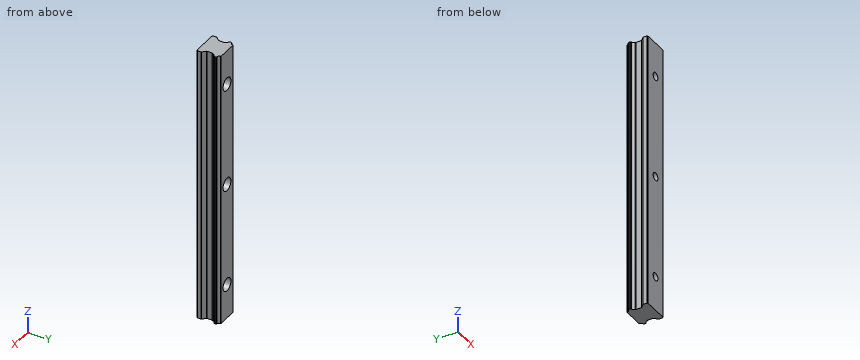
Autodesk Inventor part; units mm, degrees
ref_plane "to_block_1_XY" through (0, 13, 0) normal (0, 0, -1) x (1, 0, 0)
ref_plane "to_block_1_YZ" through (0, 13, 0) normal (1, 0, 0) x (0, -1, 0)
ref_plane "to_block_1_ZX" through (0, 13, 0) normal (0, -1, 0) x (0, 0, -1)
sketch "Sketch_2" plane through (0, 0, 0) normal (0, 0, 1) x (1, 0, 0)
  line L0 (-7.5, 10.787) -> (-7.5, 10.313)
  line L1 (-7.5, 10.313) -> (-7.2658, 9.8108)
  arc A0 (-7.2658, 9.8108) -> (-7.0326, 9.6401) centre (-6.9939, 9.9376) ccw
  arc A1 (-5.7891, 8.3153) -> (-7.0326, 9.6401) centre (-7.217, 8.221) ccw
  arc A2 (-5.7891, 8.3153) -> (-5.7019, 8.1229) centre (-5.4898, 8.335) ccw
  line L2 (-5.7019, 8.1229) -> (-5.5879, 8.0089)
  arc A3 (-5.5, 7.7967) -> (-5.5879, 8.0089) centre (-5.8, 7.7967) ccw
  line L3 (-5.5, 7.7967) -> (-5.5, 4.8243)
  arc A4 (-5.5879, 4.6121) -> (-5.5, 4.8243) centre (-5.8, 4.8243) ccw
  line L4 (-5.5879, 4.6121) -> (-7.4121, 2.7879)
  arc A5 (-7.4121, 2.7879) -> (-7.5, 2.5757) centre (-7.2, 2.5757) ccw
  line L5 (-7.5, 2.5757) -> (-7.5, 0.5)
  line L6 (-7.5, 0.5) -> (-7, 0)
  line L7 (-7, 0) -> (7, 0)
  line L8 (7, 0) -> (7.5, 0.5)
  line L9 (7.5, 0.5) -> (7.5, 2.5757)
  arc A6 (7.5, 2.5757) -> (7.4121, 2.7879) centre (7.2, 2.5757) ccw
  line L10 (7.4121, 2.7879) -> (5.5879, 4.6121)
  arc A7 (5.5, 4.8243) -> (5.5879, 4.6121) centre (5.8, 4.8243) ccw
  line L11 (5.5, 4.8243) -> (5.5, 7.7967)
  arc A8 (5.5879, 8.0089) -> (5.5, 7.7967) centre (5.8, 7.7967) ccw
  line L12 (5.5879, 8.0089) -> (5.7019, 8.1229)
  arc A9 (5.7019, 8.1229) -> (5.7891, 8.3153) centre (5.4898, 8.335) ccw
  arc A10 (7.0326, 9.6401) -> (5.7891, 8.3153) centre (7.217, 8.221) ccw
  arc A11 (7.0326, 9.6401) -> (7.2658, 9.8108) centre (6.9939, 9.9376) ccw
  line L13 (7.2658, 9.8108) -> (7.5, 10.313)
  line L14 (7.5, 10.313) -> (7.5, 10.787)
  line L15 (7.5, 10.787) -> (7.2653, 11.2903)
  arc A12 (7.2653, 11.2903) -> (7.0322, 11.461) centre (6.9934, 11.1635) ccw
  arc A13 (5.7938, 12.7312) -> (7.0322, 11.461) centre (7.217, 12.88) ccw
  arc A14 (5.7938, 12.7312) -> (5.4954, 13) centre (5.4954, 12.7) ccw
  line L16 (5.4954, 13) -> (-5.4954, 13)
  arc A15 (-5.4954, 13) -> (-5.7938, 12.7312) centre (-5.4954, 12.7) ccw
  arc A16 (-7.0322, 11.461) -> (-5.7938, 12.7312) centre (-7.217, 12.88) ccw
  arc A17 (-7.0322, 11.461) -> (-7.2653, 11.2903) centre (-6.9934, 11.1635) ccw
  line L17 (-7.2653, 11.2903) -> (-7.5, 10.787)
extrude "Extrusion1" add sketch "Sketch_2" along normal mid plane 160
sketch "Sketch2" plane through (-5.4954, 13, 80) normal (0, 1, 0) x (1, 0, 0)
  point P0 (5.4954, 20)
hole "Hole1" at (0, 13, 60) direction (0, -1, 0) diameter 4.5 depth 13 counterbore diameter 7.5 counterbore depth 6
pattern_linear "Rectangular Pattern1" count 3 spacing 60 along (0, 0, -1) of "Hole1"
ref_plane "to_block_1_XY" through (0, 13, 0) normal (0, 0, -1) x (1, 0, 0)
ref_plane "to_block_1_YZ" through (0, 13, 0) normal (1, 0, 0) x (0, -1, 0)
ref_plane "to_block_1_ZX" through (0, 13, 0) normal (0, -1, 0) x (0, 0, -1)
properties part number "C-SXR24-160_r"
The model under review builds one solid part; all positions refer to its coordinate system, in mm. Round coordinates to 2 decimals unless told otherwise and drop trailing zeros. Write each loop counter-clockwise with the first axis right and the second up, starting at its lowest first coordinate (ties: lowest second). Pieces come first, ordered by that corner, then holes. Notation, with made-up numbers: (36.5, -6) - (44.5, -6) arc R23 ccw to (44.5, 21) - close; hole circle Ø7 at (15, 56.5). An arc over 180 degrees is marked (long way). One line per question, with ' | ' between items.
Item 1: To check wall thickness, follow probe 1 along Z at (x, y) = (0, 1.75); probe 2 along Z at (x, y) = (0, 9.65); probe 3 along X at (y, z) = (2.75, 0). State the ranges of each line that lie inside material, in increasing order.
Resolved:
probe 1: z = -80 to -62.25, -57.75 to -2.25, 2.25 to 57.75, 62.25 to 80 | probe 2: z = -80 to -63.75, -56.25 to -3.75, 3.75 to 56.25, 63.75 to 80 | probe 3: x = -7.44 to -2.25, 2.25 to 7.44
Item 2: For P1, Ø5, axis at y = 3.5, z = 6, coming from the +X side; P2, Ø2.5, axis at y = 6.5, z = -3.5, coming from the +X side; P3, Ø7, axis at x = 0, z = 60, coming from the +Y side; P4, Ø0.9, axis at y = 7, z = -34.5, coming from the -X side, all flat-tipped, find the tip position at first contact; note any pin that passes through.
Resolved:
P1: stops at x = 7.5 | P2: stops at x = 5.5 | P3: stops at y = 7 | P4: stops at x = -5.5
Item 3: Add section A-A, the plane x = 0. Give the boundary of the cut face in (y, z), then the cut area to 3 significant figures.
Resolved:
outline: (0, -80) - (13, -80) - (13, -63.75) - (7, -63.75) - (7, -62.25) - (0, -62.25) - close; (0, -57.75) - (7, -57.75) - (7, -56.25) - (13, -56.25) - (13, -3.75) - (7, -3.75) - (7, -2.25) - (0, -2.25) - close; (0, 2.25) - (7, 2.25) - (7, 3.75) - (13, 3.75) - (13, 56.25) - (7, 56.25) - (7, 57.75) - (0, 57.75) - close; (0, 62.25) - (7, 62.25) - (7, 63.75) - (13, 63.75) - (13, 80) - (0, 80) - close | area: 1,850 mm2
